```python
from build123d import *

# Parameters (mm, degrees)
SKETCH_1_W          = 105
SKETCH_1_H          = 50
EXTRUDE_1_DEPTH     = 2
SKETCH_6_W          = 2
SKETCH_6_H          = 50
EXTRUDE_3_DEPTH     = 6
SKETCH_7_R          = 1.5
CUT_EXTRUDE_3_DEPTH = 6
SKETCH_8_R          = 1.5
CUT_EXTRUDE_4_DEPTH = 100


with BuildPart() as part:
    # 草图1 → 凸台-拉伸1 (new body)
    with BuildSketch(Plane(origin=(0, 0, 0), x_dir=(1, 0, 0), z_dir=(0, 1, 0))):
        Rectangle(SKETCH_1_W, SKETCH_1_H)
    extrude(amount=EXTRUDE_1_DEPTH)

    # 草图6 → 凸台-拉伸3 (add)
    with BuildSketch(Plane(origin=(0, 2, 0), x_dir=(1, 0, 0), z_dir=(0, 1, 0))):
        with Locations((-46.5, 0)):
            Rectangle(SKETCH_6_W, SKETCH_6_H)
        with Locations((46.5, 0)):
            Rectangle(SKETCH_6_W, SKETCH_6_H)
    extrude(amount=EXTRUDE_3_DEPTH)

    # 草图7 → 切除-拉伸3 (cut)
    with BuildSketch(Plane(origin=(0, 2, 0), x_dir=(1, 0, 0), z_dir=(0, 1, 0))):
        with Locations(Location((-50, 14, 0), (0, 0, 270))):
            Circle(SKETCH_7_R)
        with Locations(Location((-50, -14, 0), (0, 0, 270))):
            Circle(SKETCH_7_R)
        with Locations(Location((50, 14, 0), (0, 0, 270))):
            Circle(SKETCH_7_R)
        with Locations(Location((50, -14, 0), (0, 0, 270))):
            Circle(SKETCH_7_R)
        with Locations(Location((0, 14, 0), (0, 0, 270))):
            Circle(SKETCH_7_R)
        with Locations(Location((0, -14, 0), (0, 0, 270))):
            Circle(SKETCH_7_R)
    extrude(amount=-CUT_EXTRUDE_3_DEPTH, mode=Mode.SUBTRACT)

    # 草图8 → 切除-拉伸4 (cut)
    with BuildSketch(Plane.ZY.offset(47.5)):
        with Locations((-22.5, 5)):
            Circle(SKETCH_8_R)
        with Locations((22.5, 5)):
            Circle(SKETCH_8_R)
    extrude(amount=-CUT_EXTRUDE_4_DEPTH, mode=Mode.SUBTRACT)


solid = part.part
```
Input: part model. Units: mm. Frame: model coordinates. A direction names the side the tool comes from. Round coordinates to 2 decimals unless told otherwise and drop trailing zeros. Order: outer loops, then holes, each group sorted by start corner. A loop starts at its lowest first (then second) coordinate and runs counter-clockwise, first axis right, second up. Notation, with made-up numbers: (7.5, 24) - (31.5, 24) arc R19 ccw to (31.5, 41) - close; hole circle Ø4 at (42.5, 27). An arc over 180 degrees is marked (long way). One line per question, with ' | ' between items. Start each with the question number.
1) Set-up query: faces 4 (the flat face through (45.5, 5, 0)), 5 (the flat face through (47.5, 5, 0)), 6 (the cylindrical face through (0.07, 1.01, 12.5)), 7 (the flat face through (-47.5, 5, 0)). Return all of +Z, -Z, +X, -X, +Y, -Y with unobstructed straight access to the full face (end or side cutting, diameter ignored); none if empty.
2) Ray query, probe 1 along X at (y, z) = (1.5, -14); probe 2 along X at (y, z) = (5, 5); probe 3 along Y at (x, z) = (21.5, 0). Return the intervals inside material, ascending.
3) Cut plane C-C, the plane z = -14. Return the cut outline in (x, y).
4) Cut plane D-D, the plane x = 50. Return the cut outline in (y, z).
5) Cut plane A-A, the plane y = 5. Return the cut outline in (x, z), then the cut area to 3 significant figures.
6) Cut plane B-B, the plane z = -22.5. Return the cut outline in (x, y), then the cut area to 3 significant figures.
7) Pull-direction query (Y, two-part tool) for faces 1 (the cylindrical face through (-51.464, 1.014, 13.675)), 2 (the cylindrical face through (46, 5, 21)), 3 (the flat face through (-1, 2, 0)); classes: +Y half, -Y half, draft (parallel to the pull), parting line (faces both ways), or undercut.
8) Contact query for flat-ended pins moving along their axis: P1, Ø1.5, axis at y = 6.5, z = 6, coming from the -X side; P2, Ø2, axis at y = 6, z = -5.5, coming from the +X side; P3, Ø4, axis at x = 39, z = -14, coming from the +Y side. Output: stop coordinate, or through.
Worked out:
1) face 4: +Z, -Z, +Y | face 5: +Z, -Z, +X, +Y | face 6: +Y, -Y | face 7: +Z, -Z, -X, +Y
2) probe 1: x = -52.5 to -51.5, -48.5 to -1.5, 1.5 to 48.5, 51.5 to 52.5 | probe 2: x = -47.5 to -45.5, 45.5 to 47.5 | probe 3: y = 0 to 2
3) outline: (-52.5, 0) - (-51.5, 0) - (-51.5, 2) - (-52.5, 2) - close; (-48.5, 0) - (-1.5, 0) - (-1.5, 2) - (-45.5, 2) - (-45.5, 8) - (-47.5, 8) - (-47.5, 2) - (-48.5, 2) - close; (1.5, 0) - (48.5, 0) - (48.5, 2) - (47.5, 2) - (47.5, 8) - (45.5, 8) - (45.5, 2) - (1.5, 2) - close; (51.5, 0) - (52.5, 0) - (52.5, 2) - (51.5, 2) - close
4) outline: (0, -25) - (2, -25) - (2, -15.5) - (0, -15.5) - close; (0, -12.5) - (2, -12.5) - (2, 12.5) - (0, 12.5) - close; (0, 15.5) - (2, 15.5) - (2, 25) - (0, 25) - close
5) outline: (-47.5, -25) - (-45.5, -25) - (-45.5, -24) - (-47.5, -24) - close; (-47.5, -21) - (-45.5, -21) - (-45.5, 21) - (-47.5, 21) - close; (-47.5, 24) - (-45.5, 24) - (-45.5, 25) - (-47.5, 25) - close; (45.5, -25) - (47.5, -25) - (47.5, -24) - (45.5, -24) - close; (45.5, -21) - (47.5, -21) - (47.5, 21) - (45.5, 21) - close; (45.5, 24) - (47.5, 24) - (47.5, 25) - (45.5, 25) - close | area: 176 mm^2
6) outline: (-52.5, 0) - (52.5, 0) - (52.5, 2) - (47.5, 2) - (47.5, 3.5) - (45.5, 3.5) - (45.5, 2) - (-45.5, 2) - (-45.5, 3.5) - (-47.5, 3.5) - (-47.5, 2) - (-52.5, 2) - close; (-47.5, 6.5) - (-45.5, 6.5) - (-45.5, 8) - (-47.5, 8) - close; (45.5, 6.5) - (47.5, 6.5) - (47.5, 8) - (45.5, 8) - close | area: 222 mm^2
7) face 1: draft | face 2: undercut | face 3: +Y half
8) P1: stops at x = -47.5 | P2: stops at x = 47.5 | P3: stops at y = 2
